Answer from the drawing. Dimensions are ordinates in mm from the lowest x, y and z of the part. Give positions to 0.01 mm unless a question says otherwise; leave off trailing zeros. Loops run counter-clockwise (first coordinate to the right, second up) from the corner with the lowest first, then second, coordinate; pieces in that order, holes last. Notation, with made-up numbers: (57, 2.25) -> (62, 2.25) arc R19 ccw to (62, 20.25) -> close; hole circle Ø2 at (85.5, 68.25). An arc over 180 degrees is marked (long way). Write each question's results on one line, items separated by ' | '. Start each with the question number.
Item 1: Section A-A on y = 40 is taken. Write down the section's boundary in (x, z).
Item 2: Find the intervals of material crossed by line 1 (Z direction, x = 2.5, y = 59); line 2 (Y direction, x = 0.9, z = 43.5) (1 decimal); line 3 (Y direction, x = 0.7, z = 33.5), in increasing order.
Item 3: Section B-B on z = 24 is taken. Write down the section's boundary in (x, y).
Item 4: Each of these flat-tipped pins is pushed along its axis until it touches: P1, Ø0.8, axis at x = 2, z = 79, coming from the -Y side; P2, Ø1.5, axis at x = 0.5, z = 50, coming from the +Y side; P3, Ø0.8, axis at x = 2, y = 1, coming from the -Z side. Where does it stop, or does it pass through?
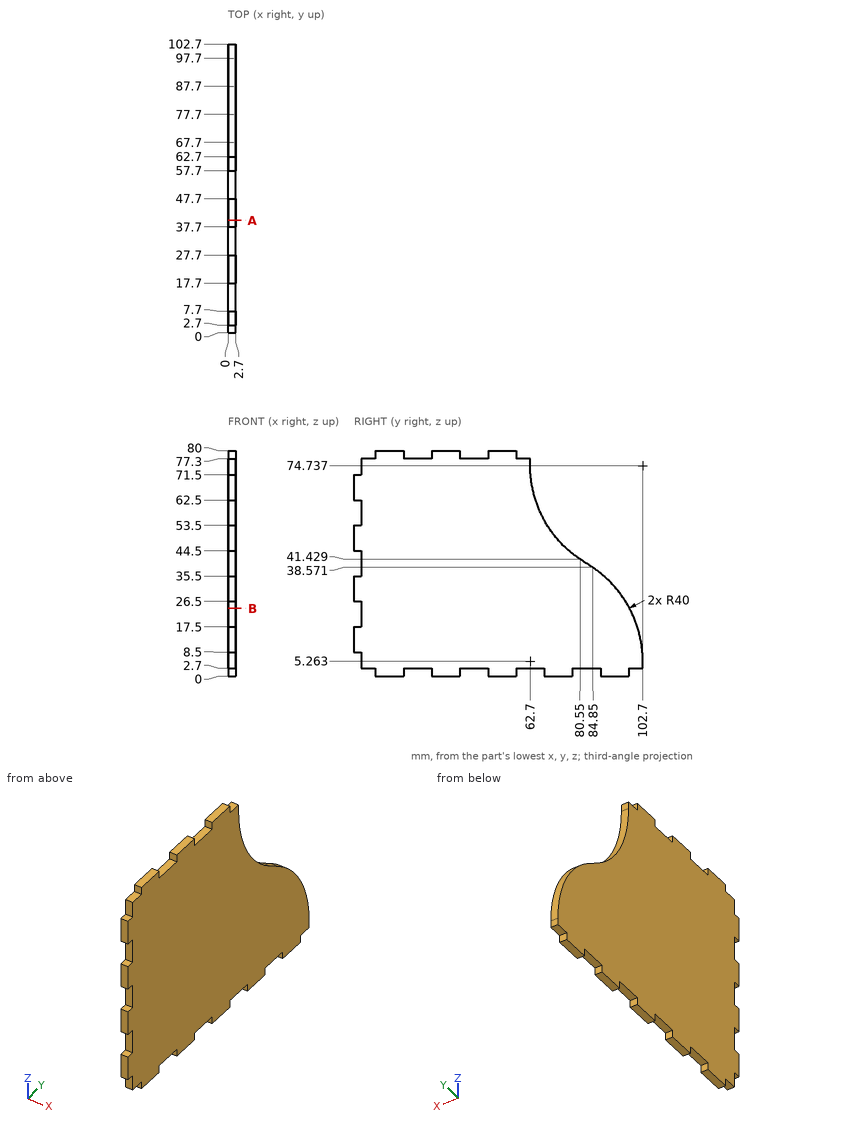
Findings:
1) outline: (0, 2.7) -> (2.7, 2.7) -> (2.7, 77.3) -> (0, 77.3) -> close
2) line 1: 2.7 to 77.3 | line 2: 2.7 to 77.7 | line 3: 0 to 91.03
3) outline: (0, 2.7) -> (2.7, 2.7) -> (2.7, 98.04) -> (0, 98.04) -> close
4) P1: y = 7.7 | P2: y = 71.87 | P3: z = 8.5
